Could you check a few things on this model? Use its own coordinates, in mm. A direction names the side the tool comes from. Give positions to 0.01 mm unless a question says otherwise; leave off trailing zeros. Write each loop counter-clockwise with the first axis right and the second up, starting at its lowest first coordinate (ties: lowest second). Pieces come first, ordered by that corner, then holes. Notation, with made-up numbers: M 81,55 L 140,55 A20 cw 140,80 Z; hole C -26,-36.5 d1. An arc over 180 degrees is marked long. Write each question's results on one line, items separated by ' | '. Start each with the question number.
from build123d import *

# Parameters (mm, degrees)
SKETCH_1_R          = 3.5
EXTRUDE_1_DEPTH     = 5
FILLET_1_R          = 2
SKETCH_2_W          = 2.6
SKETCH_2_H          = 2.6
CUT_EXTRUDE_1_DEPTH = 4
CHAMFER_1_SIZE      = 1
CHAMFER_1_SIZE2     = 2.144506921


with BuildPart() as part:
    # Эскиз1 → Бобышка-Вытянуть1 (new body)
    with BuildSketch(Plane.XY):
        Circle(SKETCH_1_R)
    extrude(amount=EXTRUDE_1_DEPTH)

    # Скругление1
    fillet_1_edges = [part.edges().sort_by_distance(p)[0] for p in [
        (-3.5, 0, 5),
    ]]
    fillet(fillet_1_edges, radius=FILLET_1_R)

    # Эскиз2 → Вырез-Вытянуть1 (cut)
    with BuildSketch(Plane(origin=(0, 0, 0), x_dir=(-1, 0, 0), z_dir=(0, 0, -1))):
        Rectangle(SKETCH_2_W, SKETCH_2_H)
    extrude(amount=-CUT_EXTRUDE_1_DEPTH, mode=Mode.SUBTRACT)

    # Фаска1
    chamfer_1_edges = [part.edges().sort_by_distance(p)[0] for p in [
        (-3.5, 0, 0),
    ]]
    chamfer_1_side = [part.faces().sort_by_distance(p)[0] for p in [
        (-3.401005051, 0, 0),
    ]]
    chamfer(chamfer_1_edges, length=CHAMFER_1_SIZE, length2=CHAMFER_1_SIZE2, reference=chamfer_1_side[0])


solid = part.part
Q1. If we section it at A-A (z = 2.6): Please give me the cut outline in (x, y), plus the area to 3 significant figures.
Q2. If we mould it in two halves opening along X, with no side actions, what happens to faces 1 (the face through (-1.3, 0, 2)), 2 (the face through (3.233, -1.341, 2.566)), 3 (the face through (0, 0, 5))? For each: pulls with the +X half, pulls with the -X half, needs draft (parallel to the pull), parting line crosses it, or undercut.
Q3. For faces 4 (the face through (2, 0, 0)), 5 (the face through (0, -1.3, 2)), which set-ups out of +Z, -Z, +X, -X, +Y, -Y let a thin tool reach every point of the face, with its end or its side?
Q4. Please list where these lines run through material, in increasing order: line 1 (Y direction, x = 0, z = 2.6); line 2 (X direction, y = 0.25, z = 1.65); line 3 (Z direction, x = 1, y = 0). Write a range as [from, to].
Q5. If we section it at B-B (z = 0.9): Please give me the cut outline in (x, y), plus the area to 3 significant figures.
Q6. I'm going to push flat-ended pins straight in: P1, Ø2, axis at x = -2.5, z = 1.5, coming from the -Y side; P2, Ø0.8, axis at x = -0.5, y = 0.5, coming from the -Z side. Where does each tip first touch, or does it pass through?
Determined:
1) outline: C 0,0 d7; hole M -1.3,-1.3 L 1.3,-1.3 L 1.3,1.3 L -1.3,1.3 Z | area: 31.7 mm²
2) face 1: undercut | face 2: parting line crosses it | face 3: needs draft
3) face 4: -Z, +X, -X, +Y, -Y | face 5: -Z
4) line 1: y = [-3.5, -1.3], [1.3, 3.5] | line 2: x = [-3.26, -1.3], [1.3, 3.26] | line 3: z = [4, 5]
5) outline: C 0,0 d5.84; hole M -1.3,-1.3 L 1.3,-1.3 L 1.3,1.3 L -1.3,1.3 Z | area: 20.0 mm²
6) P1: stops at y = -3.04 | P2: stops at z = 4
